```python
from build123d import *

# Parameters (mm, degrees)
SKETCH1_W                   = 297
SKETCH1_H                   = 210
BOSS_EXTRUDE1_DEPTH         = 2
SKETCH4_W                   = 25
SKETCH4_H                   = 12.7
BOSS_EXTRUDE2_DEPTH         = 4
M5_TAPPED_HOLE1_D           = 4.2
M5_TAPPED_HOLE1_CSINK_D     = 5.05
M5_TAPPED_HOLE1_CSINK_ANGLE = 90


with BuildPart() as part:
    # Sketch1 → Boss-Extrude1 (new body)
    with BuildSketch(Plane(origin=(0, 0, 0), x_dir=(1, 0, 0), z_dir=(0, 1, 0))):
        Rectangle(SKETCH1_W, SKETCH1_H)
    extrude(amount=BOSS_EXTRUDE1_DEPTH)

    # Sketch4 → Boss-Extrude2 (add)
    with BuildSketch(Plane(origin=(0, 2, 0), x_dir=(1, 0, 0), z_dir=(0, 1, 0))):
        with Locations((101.75, 0)):
            Rectangle(SKETCH4_W, SKETCH4_H)
        with Locations((-101.75, 0)):
            Rectangle(SKETCH4_W, SKETCH4_H)
    extrude(amount=BOSS_EXTRUDE2_DEPTH)

    # M5 Tapped Hole1 (through all)
    with Locations(Plane(origin=(0, 6, 0), x_dir=(1, 0, 0), z_dir=(0, 1, 0))):
        with Locations((-109.25, 0), (109.25, 0), (94.25, 0), (-94.25, 0)):
            CounterSinkHole(M5_TAPPED_HOLE1_D / 2, M5_TAPPED_HOLE1_CSINK_D / 2, counter_sink_angle=M5_TAPPED_HOLE1_CSINK_ANGLE)


solid = part.part
```
Read the model definition and answer for the solid it produces. Units are mm, in the model's axes. Round coordinates to 2 decimals unless told otherwise and drop trailing zeros. Loops run counter-clockwise (first coordinate to the right, second up) from the corner with the lowest first, then second, coordinate; pieces in that order, holes last. Notation, with made-up numbers: (45.5, -17.5) -> (57.5, -17.5) arc R29 ccw to (57.5, 5.5) -> close; hole circle Ø3 at (43, 29). An arc over 180 degrees is marked (long way). One line per item, written item: value.
1) Flat-ended cylindrical pins translate along their axes: P1, Ø1.2, axis at x = 101, y = 4, coming from the -Z side; P2, Ø3, axis at x = 101.5, y = 4, coming from the +Z side; P3, Ø3, axis at x = 106.5, z = -68.5, coming from the +Y side. Find the tip coordinate at first contact, or state that the pin passes through.
Answer list:
P1: stops at z = -6.35
P2: stops at z = 6.35
P3: stops at y = 2
2) A cutting plane is placed at A-A (x = 20). Determine the outline of the cut face in (y, z).
Answer list:
outline: (0, -105) -> (2, -105) -> (2, 105) -> (0, 105) -> close
3) Consider L1, parallel to Z at x = -109.25, y = 1.25; L2, parallel to Z at x = -94.25, y = 2.4; L3, parallel to Z at x = 98, y = 4.8. Determine where each line is inside the solid, lowest interval first. Write a range as [from, to].
Answer list:
L1: z = [-105, -2.1], [2.1, 105]
L2: z = [-6.35, -2.1], [2.1, 6.35]
L3: z = [-6.35, 6.35]
4) A cutting plane is placed at B-B (z = 84.5). Determine the outline of the cut face in (x, y).
Answer list:
outline: (-148.5, 0) -> (148.5, 0) -> (148.5, 2) -> (-148.5, 2) -> close
